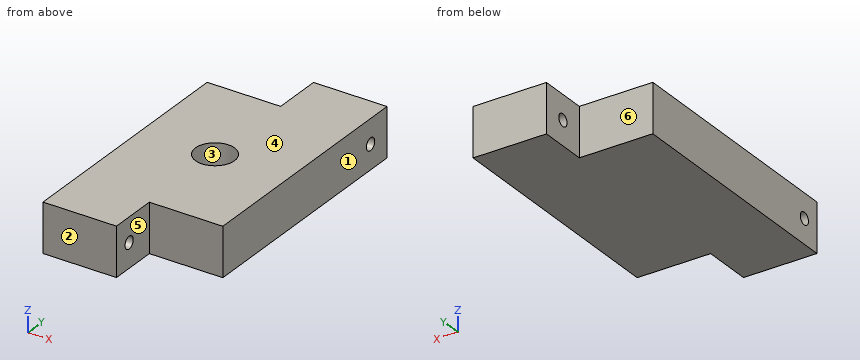
Autodesk Inventor part; units mm, degrees
ref_plane "YZ Plane" through (0, 0, 0) normal (1, 0, 0) x (0, 1, 0)
ref_plane "XZ Plane" through (0, 0, 0) normal (0, 1, 0) x (-1, 0, 0)
ref_plane "XY Plane" through (0, 0, 0) normal (0, 0, 1) x (1, 0, 0)
sketch "Sketch1" plane through (0, 0, 0) normal (0, 0, 1) x (1, 0, 0)
  line L0 (-19.05, -38.1) -> (19.05, -38.1)
  line L1 (19.05, -38.1) -> (19.05, 38.1)
  line L2 (19.05, 38.1) -> (-19.05, 38.1)
  line L3 (-19.05, 38.1) -> (-19.05, -38.1)
  line L4 (-19.05, -38.1) -> (19.05, 38.1) construction
  line L5 (19.05, -38.1) -> (-19.05, 38.1) construction
  point P0 (0, 0)
  dimension "d0" = 38.1
  dimension "d1" = 76.2
extrude "Extrusion1" add sketch "Sketch1" along normal blind 12.7
sketch "Sketch2" plane through (0, 0, 12.7) normal (0, 0, 1) x (1, 0, 0)
  line L0 (-19.05, 38.1) -> (0, 38.1)
  line L1 (0, 38.1) -> (0, 25.4)
  line L2 (0, 25.4) -> (-19.05, 25.4)
  line L3 (-19.05, 25.4) -> (-19.05, 38.1)
  point P0 (0, 0)
  dimension "d4" = 19.05
  dimension "d5" = 12.7
extrude "Extrusion2" cut sketch "Sketch2" against normal blind 12.7
sketch "Sketch3" plane through (0, 0, 12.7) normal (0, 0, 1) x (1, 0, 0)
  line L0 (19.05, -38.1) -> (0, -38.1)
  line L1 (0, -38.1) -> (0, -25.4)
  line L2 (0, -25.4) -> (19.05, -25.4)
  line L3 (19.05, -25.4) -> (19.05, -38.1)
  point P0 (0, 0)
  dimension "d8" = 19.05
  dimension "d9" = 12.7
extrude "Extrusion3" cut sketch "Sketch3" against normal blind 12.7
sketch "Sketch4" plane through (0, 0, 12.7) normal (0, 0, 1) x (1, 0, 0)
  circle A0 centre (0, 0) radius 5.08
  dimension "d12" = 10.16
extrude "Extrusion4" cut sketch "Sketch4" against normal blind 6.35
sketch "Sketch5" plane through (19.05, 38.1, 12.7) normal (1, 0, 0) x (0, 0, -1)
  line L0 (12.7, -76.2) -> (12.7, 0)
  line L1 (12.7, 0) -> (0, 0)
  line L2 (0, -63.5) -> (0, 0)
  line L3 (0, -12.7) -> (12.7, -12.7)
  circle A0 centre (6.35, -6.35) radius 1.5875
  point P0 (12.7, -63.5)
  point P1 (12.7, -38.1)
  dimension "d16" = 3.175
  dimension "d17" = 6.35
  dimension "d18" = 6.35
  dimension "d19" = 6.35
  dimension "d20" = 6.35
extrude "Extrusion5" cut sketch "Sketch5" against normal blind 19.05 contours A0
sketch "Sketch9" plane through (-19.05, -38.1, 0) normal (-1, 0, 0) x (0, 0, 1)
  line L0 (0, 0) -> (12.7, 0)
  line L1 (12.7, 63.5) -> (12.7, 0)
  line L2 (12.7, 9.7791) -> (0, 9.7791)
  circle A0 centre (6.35, 4.8896) radius 1.5875
  point P0 (0, 38.1)
  dimension "d34" = 3.175
  dimension "d35" = 6.35
  dimension "d36" = 4.8896
  dimension "d37" = 4.8896
extrude "Extrusion9" cut sketch "Sketch9" against normal blind 19.05
equation "\"d17\" = d18"
equation "\"d19\" = d20"
equation "\"d36\" = d37"
properties part number "MotorMount"
Here's how the part is built. I have some questions about the finished solid (model axes, mm). Face numbers are marked on the shaded views. A direction names the side the tool comes from. Give positions to 0.01 mm unless a question says otherwise; leave off trailing zeros. Write each loop counter-clockwise with the first axis right and the second up, starting at its lowest first coordinate (ties: lowest second). Pieces come first, ordered by that corner, then holes. Notation, with made-up numbers: (-24.75, -14) -> (-14.75, -14) arc R28 cw to (-14.75, 19) -> close; hole circle Ø9 at (84.25, 30.25). An arc over 180 degrees is marked (long way). Use one line per item in the form item = value. Start each with the question number.
1. Imagine slicing it at A-A on z = 10.5. List the corners of the cut face in (x, y) for me, plus the area to 3 significant figures.
2. If I drill on L1, parallel to Y at x = 12.75, z = 6.35; L2, parallel to Y at x = -11.5, z = 6.35; L3, parallel to X at y = -2.5, z = 11, over which ranges is the centre line in solid material (lowest first)?
3. On a 3-axis mill with a long thin cutter (end or side, diameter ignored), from which of +Z, -Z, +X, -X, +Y, -Y can I reach the whole of each face in a straight line? I mean the marked faces 4, 5 and 6. Say none if no direction works.
4. Imagine slicing it at B-B on y = 31.75. List the corners of the cut face in (x, z) for me.
5. Will these pins go through, and if not, where does the flat tip stop? pin 1 Ø4 at (y, z) = (-34.5, 6.5) entering from +X; pin 2 Ø5 at (x, y) = (-1, -0.5) entering from +Z; pin 3 Ø4 at (y, z) = (31.75, 6.35) entering from -X.
6. Thinking about a two-plate mould opening in Y: for the marked faces 1, 2 and 3, which applies, +Y half, -Y half, draft (parallel to the pull), parting line (faces both ways), or undercut?
7. Imagine slicing it at D-D on z = 3.75. List the corners of the cut face in (x, y) for me, plus the area to 3 significant figures.
Entries:
q1.outline = (-19.05, -38.1) -> (0, -38.1) -> (0, -25.4) -> (19.05, -25.4) -> (19.05, 38.1) -> (0, 38.1) -> (0, 25.4) -> (-19.05, 25.4) -> close; hole circle Ø10.16 at (0, 0)
q1.area = 2,340 mm²
q2.L1 = -25.4 to 30.16, 33.34 to 38.1
q2.L2 = -38.1 to -34.8, -31.62 to 25.4
q2.L3 = -19.05 to -4.42, 4.42 to 19.05
q3.face_4 = +Z, +X, -X, +Y, -Y
q3.face_5 = +Z, -Z, +X, -Y
q3.face_6 = +Z, -Z, -X, +Y
q4.outline = (0, 0) -> (19.05, 0) -> (19.05, 4.76) -> (0, 4.76) -> close; (0, 7.94) -> (19.05, 7.94) -> (19.05, 12.7) -> (0, 12.7) -> close
q5.pin_1 = 0
q5.pin_2 = 6.35
q5.pin_3 = 0
q6.face_1 = draft
q6.face_2 = -Y half
q6.face_3 = undercut
q7.outline = (-19.05, -38.1) -> (0, -38.1) -> (0, -25.4) -> (19.05, -25.4) -> (19.05, 38.1) -> (0, 38.1) -> (0, 25.4) -> (-19.05, 25.4) -> close
q7.area = 2,420 mm²
